```python
from build123d import *

# Parameters (mm, degrees)
SKETCH1_W               = 165.1
SKETCH1_H               = 101.6
BOSS_EXTRUDE1_DEPTH     = 7.62
SKETCH2_W               = 160.02
SKETCH2_H               = 96.52
CUT_EXTRUDE1_DEPTH      = 2.54
BOSS_EXTRUDE2_START     = -7.62
BOSS_EXTRUDE2_DEPTH     = 0.635
SKETCH4_R               = 1.905
CUT_EXTRUDE2_DEPTH      = 103.203442334
MIRROR2_START           = -7.62
MIRROR2_COPY_1_DEPTH    = 0.635
MIRROR2_COPY_2_SKETCH_R = 1.905
MIRROR2_COPY_2_DEPTH    = 103.203442334


with BuildPart() as part:
    # Sketch1 → Boss-Extrude1 (new, symmetric)
    with BuildSketch(Plane.XY):
        Rectangle(SKETCH1_W, SKETCH1_H)
    extrude(amount=BOSS_EXTRUDE1_DEPTH, both=True)

    # Sketch2 → Cut-Extrude1 (cut)
    with BuildSketch(Plane.XY.offset(7.62)):
        Rectangle(SKETCH2_W, SKETCH2_H)
    extrude(amount=-CUT_EXTRUDE1_DEPTH, mode=Mode.SUBTRACT)

    # Sketch3 → Boss-Extrude2 (add, symmetric)
    with BuildSketch(Plane(origin=(0, 0, -7.62), x_dir=(-1, 0, 0), z_dir=(0, 0, -1)).offset(BOSS_EXTRUDE2_START)):
        with BuildLine():
            Line((-82.55, 55.88), (-82.55, 50.8))
            Line((-82.55, 50.8), (-74.93, 50.8))
            Line((-74.93, 50.8), (-74.93, 55.88))
            ThreePointArc((-74.93, 55.88), (-78.74, 59.69), (-82.55, 55.88))
        make_face()
    boss_extrude2 = extrude(amount=BOSS_EXTRUDE2_DEPTH, both=True)

    # Sketch4 → Cut-Extrude2 (cut, through all)
    with BuildSketch(Plane.XY.offset(0.635)):
        with Locations((78.74, 55.88)):
            Circle(SKETCH4_R)
    cut_extrude2 = extrude(amount=-CUT_EXTRUDE2_DEPTH, mode=Mode.SUBTRACT)

    # Mirror1: Boss-Extrude2, Cut-Extrude2 across plane
    add(boss_extrude2.mirror(Plane.ZX))
    add(cut_extrude2.mirror(Plane.ZX), mode=Mode.SUBTRACT)

    # Mirror2: Boss-Extrude2, Cut-Extrude2 across plane
    add(boss_extrude2.mirror(Plane(origin=(0, 0, 0), x_dir=(0, 0, 1), z_dir=(1, 0, 0))))
    add(cut_extrude2.mirror(Plane(origin=(0, 0, 0), x_dir=(0, 0, 1), z_dir=(1, 0, 0))), mode=Mode.SUBTRACT)

    # Mirror2 copy 1 sketch → Mirror2 copy 1 (add, symmetric)
    with BuildSketch(Plane(origin=(0, 0, -7.62), x_dir=(1, 0, 0), z_dir=(0, 0, -1)).offset(MIRROR2_START)):
        with BuildLine():
            Line((-82.55, 55.88), (-82.55, 50.8))
            Line((-82.55, 50.8), (-74.93, 50.8))
            Line((-74.93, 50.8), (-74.93, 55.88))
            ThreePointArc((-74.93, 55.88), (-78.74, 59.69), (-82.55, 55.88))
        make_face()
    extrude(amount=MIRROR2_COPY_1_DEPTH, both=True)

    # Mirror2 copy 2 sketch → Mirror2 copy 2 (cut, through all)
    with BuildSketch(Plane(origin=(0, 0, 0.635), x_dir=(-1, 0, 0), z_dir=(0, 0, 1))):
        with Locations((78.74, 55.88)):
            Circle(MIRROR2_COPY_2_SKETCH_R)
    extrude(amount=-MIRROR2_COPY_2_DEPTH, mode=Mode.SUBTRACT)


solid = part.part
```
Build history of the part. All positions in model axes, mm. A direction names the side the tool comes from. Give positions to 0.01 mm unless a question says otherwise; leave off trailing zeros. Loops run counter-clockwise (first coordinate to the right, second up) from the corner with the lowest first, then second, coordinate; pieces in that order, holes last.
Item 1: Drill centre lines: line 1 (X direction, y = -55.88, z = -0.3) (3 decimals); line 2 (Y direction, x = -78.74, z = 0.15) (3 decimals); line 3 (X direction, y = 33.5, z = 5.75). Where is each one in solid material? Low to high.
Answers follow:
line 1: x = -82.55 to -80.645, -76.835 to -74.93, 74.93 to 76.835, 80.645 to 82.55
line 2: y = -59.69 to -57.785, -53.975 to 53.975, 57.785 to 59.69
line 3: x = -82.55 to -80.01, 80.01 to 82.55
Item 2: Pull direction X, two halves, no side cores. Call faces 6 (the face through (-79, -53, 0.635)), 7 (the face through (82.55, -1, 0)), 8 (the face through (78.33, 54.02, 0.01)): released by +X, released by -X, zero draft, split by the parting line, or undercut.
Answers follow:
face 6: zero draft
face 7: released by +X
face 8: undercut
Item 3: Which spindle directions (+Z, -Z, +X, -X, +Y, -Y) get a long thin tool onto all of the face, cutting with end or side? Do faces 1 (the face through (79, -53, -0.635)), 2 (the face through (-1, 1, 5.08)), 3 (the face through (-79, 53, -0.635)), 4 (the face through (79, 53, 0.635)), 5 (the face through (79, -53, 0.635)). Say none if no direction does.
Answers follow:
face 1: -Z, +X, -X, -Y
face 2: +Z
face 3: -Z, +X, -X, +Y
face 4: +Z, +X, -X, +Y
face 5: +Z, +X, -X, -Y
Item 4: Slice it at B-B, the plane x = 21.5. List the corners of the cut face in (y, z), and give its area (3 significant figures).
Answers follow:
outline: (-50.8, -7.62) - (50.8, -7.62) - (50.8, 7.62) - (48.26, 7.62) - (48.26, 5.08) - (-48.26, 5.08) - (-48.26, 7.62) - (-50.8, 7.62) - close
area: 1,300 mm2
Item 5: Flat gauge pins, fed straight in: pin 1 (8 mm diameter, centred on x = -32.5, z = 4, fed in from +Y); pin 2 (4 mm diameter, centred on x = 64, y = -12.5, fed in from +Z); pin 3 (2.5 mm diameter, centred on x = 78.5, y = -54, fed in from +Z) (3 decimals). Where does each tip first touch, or does it go through?
Answers follow:
pin 1: stops at y = 50.8
pin 2: stops at z = 5.08
pin 3: stops at z = 0.635
Item 6: Slice it at A-A, the plane y = 42. List the corners of the cut face in (x, z).
Answers follow:
outline: (-82.55, -7.62) - (82.55, -7.62) - (82.55, 7.62) - (80.01, 7.62) - (80.01, 5.08) - (-80.01, 5.08) - (-80.01, 7.62) - (-82.55, 7.62) - close
